Autodesk Inventor part; units mm, degrees
ref_plane "YZ Plane" through (0, 0, 0) normal (1, 0, 0) x (0, 1, 0)
ref_plane "XZ Plane" through (0, 0, 0) normal (0, 1, 0) x (-1, 0, 0)
ref_plane "XY Plane" through (0, 0, 0) normal (0, 0, 1) x (1, 0, 0)
ref_plane "Work Plane1" through (0, 0, 35) normal (0, 0, 1) x (1, 0, 0)
sketch "Sketch1" plane through (0, 0, 35) normal (0, 0, 1) x (1, 0, 0)
  circle A0 centre (12.5, 45.6) radius 1.5
  circle A1 centre (19.5, 27) radius 1.5
  circle A2 centre (5.5, 27) radius 1.5
  circle A3 centre (12.5, 20) radius 1.5
  circle A4 centre (12.5, 34) radius 1.5
  circle A5 centre (12.5, 8.4) radius 1.5
  circle A6 centre (12.5, 27) radius 4
  line L0 (0, 0) -> (25, 0)
  line L1 (25, 0) -> (25, 54)
  line L2 (0, 54) -> (25, 54)
  line L3 (0, 0) -> (0, 54)
  line L4 (25, 54) -> (0, 54)
  line L5 (0, 54) -> (0, 0)
  line L6 (0, 0) -> (25, 0)
  line L7 (25, 0) -> (25, 54)
  circle A7 centre (12.5, 45.6) radius 1.5
  circle A8 centre (12.5, 27) radius 4
  circle A9 centre (19.5, 27) radius 1.5
  circle A10 centre (12.5, 34) radius 1.5
  circle A11 centre (12.5, 20) radius 1.5
  circle A12 centre (5.5, 27) radius 1.5
  circle A13 centre (12.5, 8.4) radius 1.5
extrude "Extrusion1" add sketch "Sketch1" along normal blind 5
sketch "Sketch4" plane through (0, 0, 40) normal (0, 0, 1) x (1, 0, 0)
  line L0 (25, 54) -> (0, 54)
  line L1 (0, 54) -> (0, 0)
  circle A0 centre (12.5, 45.6) radius 1.5
  line L2 (25, 0) -> (25, 54)
  line L3 (0, 0) -> (25, 0)
  line L4 (25, 54) -> (45, 54)
  line L5 (45, 54) -> (45, 74)
  line L6 (45, 74) -> (25, 74)
  line L7 (25, 74) -> (25, 54)
  line L8 (0, 54) -> (-20, 54)
  line L9 (-20, 54) -> (-20, 74)
  line L10 (-20, 74) -> (0, 74)
  line L11 (0, 74) -> (0, 54)
  line L12 (25, 0) -> (45, 0)
  line L13 (45, 0) -> (45, -20)
  line L14 (45, -20) -> (25, -20)
  line L15 (25, -20) -> (25, 0)
  line L16 (0, 0) -> (-20, 0)
  line L17 (-20, 0) -> (-20, -20)
  line L18 (-20, -20) -> (0, -20)
  line L19 (0, -20) -> (0, 0)
  line L20 (-20, 74) -> (-15, 74)
  line L21 (-15, 74) -> (-15, 69)
  line L22 (-15, 69) -> (-20, 69)
  line L23 (-20, 69) -> (-20, 74)
  line L24 (45, 74) -> (40, 74)
  line L25 (40, 74) -> (40, 69)
  line L26 (40, 69) -> (45, 69)
  line L27 (45, 69) -> (45, 74)
  line L28 (45, -20) -> (40, -20)
  line L29 (40, -20) -> (40, -15)
  line L30 (40, -15) -> (45, -15)
  line L31 (45, -15) -> (45, -20)
  line L32 (-20, -20) -> (-15, -20)
  line L33 (-15, -20) -> (-15, -15)
  line L34 (-15, -15) -> (-20, -15)
  line L35 (-20, -15) -> (-20, -20)
  line L36 (0, 0) -> (5, 0)
  line L37 (5, 0) -> (5, 5)
  line L38 (5, 5) -> (0, 5)
  line L39 (0, 5) -> (0, 0)
  line L40 (25, 0) -> (20, 0)
  line L41 (20, 0) -> (20, 5)
  line L42 (20, 5) -> (25, 5)
  line L43 (25, 5) -> (25, 0)
  line L44 (25, 54) -> (20, 54)
  line L45 (20, 54) -> (20, 49)
  line L46 (20, 49) -> (25, 49)
  line L47 (25, 49) -> (25, 54)
  line L48 (0, 54) -> (5, 54)
  line L49 (5, 54) -> (5, 49)
  line L50 (5, 49) -> (0, 49)
  line L51 (0, 49) -> (0, 54)
  line L52 (0, 5) -> (-20, -15)
  line L53 (5, 0) -> (-15, -20)
  line L54 (20, 0) -> (40, -20)
  line L55 (25, 5) -> (45, -15)
  line L56 (-20, 69) -> (0, 49)
  line L57 (-15, 74) -> (5, 54)
  line L58 (40, 74) -> (20, 54)
  line L59 (45, 69) -> (25, 49)
  circle A1 centre (-17.5, 71.5) radius 1.5
  circle A2 centre (42.5, 71.5) radius 1.5
  circle A3 centre (-17.5, -17.5) radius 1.5
  circle A4 centre (42.5, -17.5) radius 1.5
  dimension "d16" = 20
  dimension "d17" = 20
  dimension "d18" = 20
  dimension "d19" = 20
  dimension "d20" = 20
  dimension "d21" = 20
  dimension "d22" = 20
  dimension "d23" = 20
  dimension "d24" = 5
  dimension "d25" = 5
  dimension "d26" = 5
  dimension "d27" = 5
  dimension "d28" = 5
  dimension "d29" = 5
  dimension "d30" = 5
  dimension "d31" = 5
  dimension "d32" = 5
  dimension "d33" = 5
  dimension "d34" = 5
  dimension "d35" = 5
  dimension "d36" = 5
  dimension "d37" = 5
  dimension "d38" = 5
  dimension "d39" = 5
  dimension "d40" = 3
extrude "Extrusion3" add sketch "Sketch4" against normal blind 5 contours L2 L46 L45 L0 | L4 L59 L2 | L7 L58 L25 L26 L59 L4 | L0 L58 L7 | L49 L50 L1 L0 | L0 L11 L57 | L55 L12 L2 | L2 L3 L41 L42 | L26 L25 L6 L5 | L1 L56 L8 | L8 L56 L22 L21 L57 L11 | L15 L54 L3 | L12 L55 L30 L29 L54 L15 | L21 L22 L9 L10 | L13 L14 L29 L30 | L38 L37 L3 L1 | L1 L16 L52 | L53 L19 L3 | L19 L53 L33 L34 L52 L16 | L34 L33 L18 L17
sketch "Sketch5" plane through (0, 0, 40) normal (0, 0, 1) x (1, 0, 0)
  line L0 (-20, -20) -> (-15, -20)
  line L1 (-20, -15) -> (-20, -20)
  circle A0 centre (-17.5, -17.5) radius 1.5
  circle A1 centre (-17.5, 71.5) radius 1.5
  line L2 (-20, 74) -> (-20, 69)
  line L3 (-15, 74) -> (-20, 74)
  line L4 (45, 74) -> (40, 74)
  line L5 (45, 69) -> (45, 74)
  circle A2 centre (42.5, 71.5) radius 1.5
  circle A3 centre (42.5, -17.5) radius 1.5
  line L6 (40, -20) -> (45, -20)
  line L7 (45, -20) -> (45, -15)
  line L8 (-20, -20) -> (-15, -20)
  line L9 (-15, -20) -> (-15, -15)
  line L10 (-15, -15) -> (-20, -15)
  line L11 (-20, -15) -> (-20, -20)
  circle A4 centre (-17.5, -17.5) radius 1.5
  circle A5 centre (-17.5, 71.5) radius 1.5
  circle A6 centre (42.5, 71.5) radius 1.5
  circle A7 centre (42.5, -17.5) radius 1.5
  line L12 (40, -20) -> (45, -20)
  line L13 (45, -20) -> (45, -15)
  line L14 (45, -15) -> (40, -15)
  line L15 (40, -15) -> (40, -20)
  line L16 (45, 74) -> (40, 74)
  line L17 (40, 74) -> (40, 69)
  line L18 (40, 69) -> (45, 69)
  line L19 (45, 69) -> (45, 74)
  line L20 (-20, 69) -> (-15, 69)
  line L21 (-15, 69) -> (-15, 74)
  line L22 (-15, 74) -> (-20, 74)
  line L23 (-20, 74) -> (-20, 69)
  point P0 (0, 0)
extrude "Extrusion4" add sketch "Sketch5" along normal blind 20
properties part number "Face"
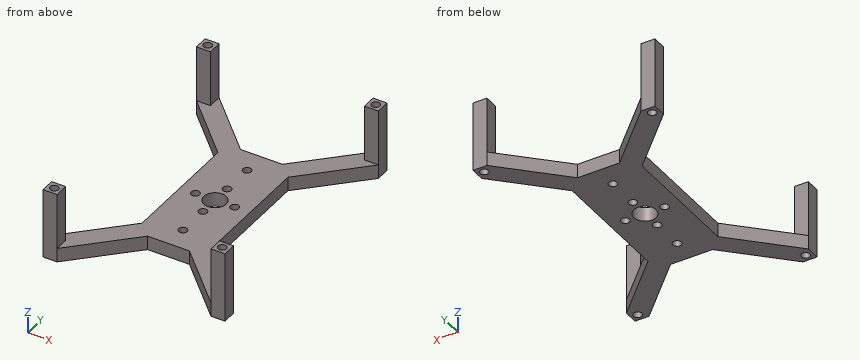
Verification items for the finished model (mm, model axes). Round coordinates to 2 decimals unless told otherwise and drop trailing zeros. Write each loop counter-clockwise with the first axis right and the second up, starting at its lowest first coordinate (ties: lowest second). Pieces come first, ordered by that corner, then holes. Notation, with made-up numbers: (58.25, -36.5) -> (108.25, -36.5) arc R20 ccw to (108.25, -31.5) -> close; hole circle Ø5 at (77.5, 54). An arc over 180 degrees is marked (long way). Write each question's results on one line, items separated by ' | '.
Q1. Go/stop test with flat-tipped pins: pin 1 Ø4 at (x, z) = (14.5, 37.5) entering from +Y; pin 2 Ø1 at (y, z) = (-10.5, 39.5) entering from +X; pin 3 Ø1 at (y, z) = (27, 37.5) entering from -X. Record where each tip stops, or that it passes through.
Derived:
pin 1: stops at y = 54 | pin 2: stops at x = 41 | pin 3: stops at x = 0
Q2. Sectioned sample at A-A, the plane z = 47.75. Record the boundary of the cut face in (x, y).
Derived:
outline: (-20, -20) -> (-15, -20) -> (-15, -15) -> (-20, -15) -> close; (-20, 69) -> (-15, 69) -> (-15, 74) -> (-20, 74) -> close; (40, -20) -> (45, -20) -> (45, -15) -> (40, -15) -> close; (40, 69) -> (45, 69) -> (45, 74) -> (40, 74) -> close; hole circle Ø3 at (-17.5, -17.5); hole circle Ø3 at (-17.5, 71.5); hole circle Ø3 at (42.5, -17.5); hole circle Ø3 at (42.5, 71.5)
Q3. Sectioned sample at C-C, the plane x = -17.5. Record the boundary of the cut face in (y, z).
Derived:
outline: (-20, 35) -> (-19, 35) -> (-19, 60) -> (-20, 60) -> close; (-16, 35) -> (-12.5, 35) -> (-12.5, 40) -> (-15, 40) -> (-15, 60) -> (-16, 60) -> close; (66.5, 35) -> (70, 35) -> (70, 60) -> (69, 60) -> (69, 40) -> (66.5, 40) -> close; (73, 35) -> (74, 35) -> (74, 60) -> (73, 60) -> close
Q4. Thickness scan on probe 1 along Y at (x, z) = (42.5, 52.5); probe 2 along Y at (x, z) = (12.5, 36.95); probe 3 along Z at (x, y) = (12, 49). Record the ranges inside material, lowest first.
Derived:
probe 1: y = -20 to -19, -16 to -15, 69 to 70, 73 to 74 | probe 2: y = 0 to 6.9, 9.9 to 18.5, 21.5 to 23, 31 to 32.5, 35.5 to 44.1, 47.1 to 54 | probe 3: z = 35 to 40
Q5. Sectioned sample at D-D, the plane y = 45.6. Record the boundary of the cut face in (x, z), and give its area (3 significant figures).
Derived:
outline: (0, 35) -> (11, 35) -> (11, 40) -> (0, 40) -> close; (14, 35) -> (25, 35) -> (25, 40) -> (14, 40) -> close | area: 110 mm²
Q6. Sectioned sample at B-B, the plane y = -17.5. Record the boundary of the cut face in (x, z).
Derived:
outline: (-20, 35) -> (-19, 35) -> (-19, 60) -> (-20, 60) -> close; (-16, 35) -> (-12.5, 35) -> (-12.5, 40) -> (-15, 40) -> (-15, 60) -> (-16, 60) -> close; (37.5, 35) -> (41, 35) -> (41, 60) -> (40, 60) -> (40, 40) -> (37.5, 40) -> close; (44, 35) -> (45, 35) -> (45, 60) -> (44, 60) -> close
